Verification items for this drawing (mm, ordinates from the low corner). A direction names the side the tool comes from. Round coordinates to 2 decimals unless told otherwise and drop trailing zeros. Loops run counter-clockwise (first coordinate to the right, second up) from the corner with the lowest first, then second, coordinate; pieces in that order, holes last. Notation, with made-up numbers: (-4.5, 31.5) - (42.5, 31.5) arc R18 cw to (42.5, 64.5) - close; hole circle Ø4 at (65.5, 82.25). An arc over 180 degrees is marked (long way). Answer in a Markdown table with one row per item. Add a question column.
(1) Access from +Z, -Z, +X, -X, +Y, -Y to the whole of each face (thin tool, end or side, straight path). Record for the marked faces 4, 5 and 6.
(2) Mould release check, pull along X, two halves, no side actions. Record for the marked faces 1, 2 and 3: +X half, -X half, draft (parallel to the pull), parting line (faces both ways), or undercut.
(3) Gauge pin test, flat ends, axial feed: pin 1 (2 mm diameter, centred on x = 1.5, y = 9, fed in from +Z); pin 2 (1.2 mm diameter, centred on y = 11, z = 2.5, fed in from +X); pin 3 (2 mm diameter, centred on y = 8.5, z = 3, fed in from -X); pin 4 (1 mm diameter, centred on x = 1, y = 9, fed in from +Z). Record the tip position at first contact, or that the pin passes through.
(4) Thickness scan on line 1 along X through (y, z) = (10.25, 2.8); line 2 along Y through (x, z) = (4, 1.2); line 3 along Z through (x, y) = (2.85, 10.5). Record the ranges inside material, lowest first.
(5) Cross-section at D-D on x = 5.5. Enter the section's corners in (y, z).
(6) Cross-section at C-C on z = 3.5. Enter the section's corners in (x, y), then the cut area to 3 significant figures.
(7) Cross-section at A-A on z = 2.3. Enter the section's corners in (x, y), then the cut area to 3 significant figures.
(8) Cross-section at B-B on y = 10.5. Enter the section's corners in (x, z), then the cut area to 3 significant figures.
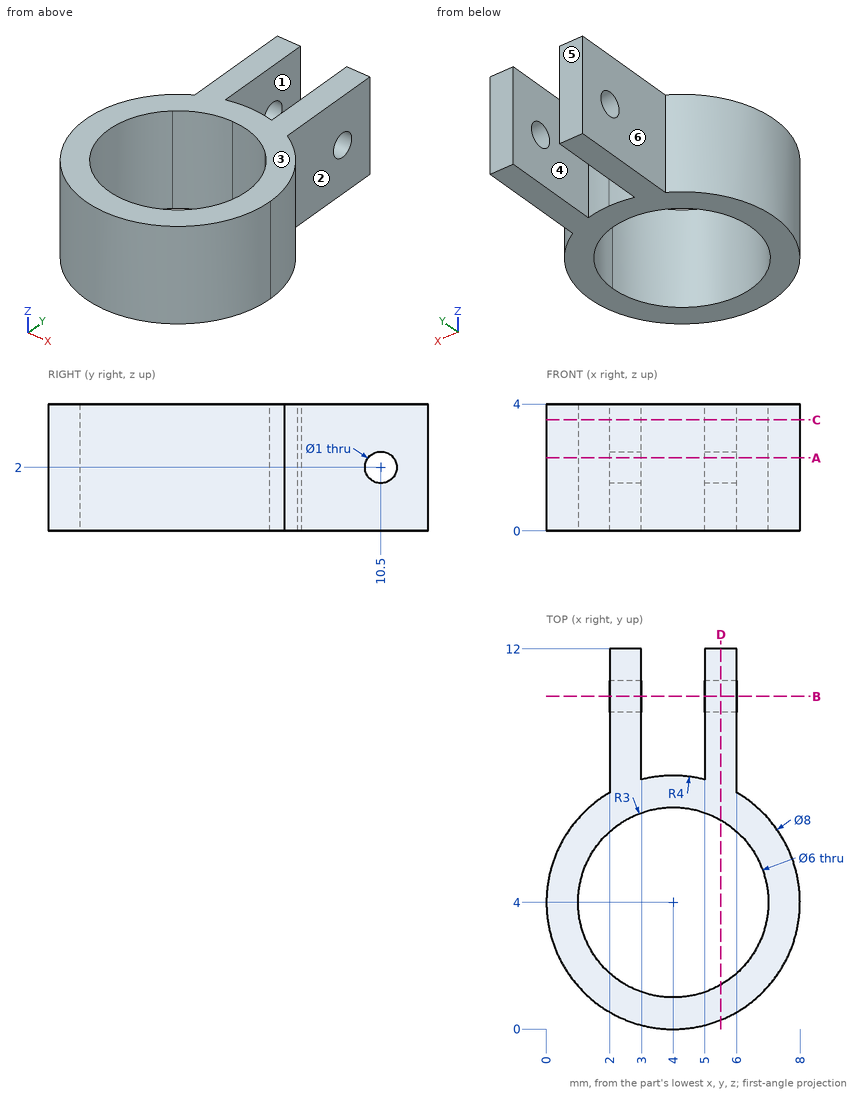
Answers:
| question | item | result |
|---|---|---|
| 1 | face 4 | +Z, -Z, +Y |
| 1 | face 5 | +Z, -Z, +X, -X, +Y |
| 1 | face 6 | +Z, -Z, -X, +Y |
| 2 | face 1 | undercut |
| 2 | face 2 | +X half |
| 2 | face 3 | draft |
| 3 | pin 1 | stops at z = 4 |
| 3 | pin 2 | stops at x = 6 |
| 3 | pin 3 | stops at x = 2 |
| 3 | pin 4 | passes through |
| 4 | line 1 | x = 2 to 3, 5 to 6 |
| 4 | line 2 | y = 0 to 1, 7 to 8 |
| 4 | line 3 | z = 0 to 1.5, 2.5 to 4 |
| 5 | outline | (0.29, 0) - (1.4, 0) - (1.4, 4) - (0.29, 4) - close; (6.6, 0) - (12, 0) - (12, 4) - (6.6, 4) - close; hole circle Ø1 at (10.5, 2) |
| 6 | outline | (2, 7.46) arc R4 ccw (long way) to (6, 7.46) - (6, 12) - (5, 12) - (5, 7.87) arc R4 ccw to (3, 7.87) - (3, 12) - (2, 12) - close; hole circle Ø6 at (4, 4) |
| 6 | area | 30.6 mm^2 |
| 7 | outline | (2, 7.46) arc R4 ccw (long way) to (6, 7.46) - (6, 10.1) - (5, 10.1) - (5, 7.87) arc R4 ccw to (3, 7.87) - (3, 10.1) - (2, 10.1) - close; (2, 10.9) - (3, 10.9) - (3, 12) - (2, 12) - close; (5, 10.9) - (6, 10.9) - (6, 12) - (5, 12) - close; hole circle Ø6 at (4, 4) |
| 7 | area | 29.0 mm^2 |
| 8 | outline | (2, 0) - (3, 0) - (3, 1.5) - (2, 1.5) - close; (2, 2.5) - (3, 2.5) - (3, 4) - (2, 4) - close; (5, 0) - (6, 0) - (6, 1.5) - (5, 1.5) - close; (5, 2.5) - (6, 2.5) - (6, 4) - (5, 4) - close |
| 8 | area | 6.00 mm^2 |
